```python
from build123d import *

# Parameters (mm, degrees)
F0_W     = 35
F0_H     = 20
F1_DEPTH = 5
F2_R     = 2.49999


# Not quite as in the source:
# - a fillet or chamfer is up to 0.001 mm smaller than in the source, because OpenCascade refuses the exact size


with BuildPart() as f1:
    # F0 (on Top) → F1 (new body)
    with BuildSketch(Plane.XY):
        Rectangle(F0_W, F0_H)
        Polygon((3, -1), (15, -1), (15, -6), (-15, -6), (-15, -1), (-3, -1), (-3, 5), (3, 5), align=None, mode=Mode.SUBTRACT)
    extrude(amount=F1_DEPTH)

    # F2 (radius 2.5 in the source; OpenCascade refuses exactly that, so slightly less here)
    f2_edges = [f1.edges().sort_by_distance(p)[0] for p in [
        (-17.5, -10, 2.5),
        (17.5, -10, 2.5),
        (0, -10, 0),
        (0, -10, 5),
    ]]
    fillet(f2_edges, radius=F2_R)


solid = f1.part
```
For this review, take the finished solid that the model builds, in its own axes (mm). A direction names the side the tool comes from. Round coordinates to 2 decimals unless told otherwise and drop trailing zeros. Order: outer loops, then holes, each group sorted by start corner. A loop starts at its lowest first (then second) coordinate and runs counter-clockwise, first axis right, second up.
Q1. Machinability: for faces 4 (the flat face through (-15, -4, 2)), 5 (the flat face through (-17.5, 1, 2)), which of the approach directions +Z, -Z, +X, -X, +Y, -Y give a long, thin tool a straight path to every point of the face, cutting with its end or side? Answer none if there is none.
Findings below:
face 4: +Z, -Z
face 5: +Z, -Z, -X, +Y, -Y
Q2. We need section D-D, the plane y = 1.75. Give the boundary of the cut face in (x, z).
Findings below:
outline: (-17.5, 0) - (-3, 0) - (-3, 5) - (-17.5, 5) - close; (3, 0) - (17.5, 0) - (17.5, 5) - (3, 5) - close
Q3. We need section C-C, the plane z = 4. Give the boundary of the cut face in (x, y).
Findings below:
outline: (-17.5, -7.5) arc R2.5 ccw to (-16.5, -9.5) - (16.5, -9.5) arc R2.5 ccw to (17.5, -7.5) - (17.5, 10) - (-17.5, 10) - close; hole (-15, -6) - (15, -6) - (15, -1) - (3, -1) - (3, 5) - (-3, 5) - (-3, -1) - (-15, -1) - close
Q4. Mouldability with a two-part tool opening along Y and no side actions: class faces 1 (the flat face through (-0.2, 5.3, 0)), 2 (the cylindrical face through (0.245, -9.287, 4.248)), 3 (the flat face through (-9, -1, 2)) as pulls with the +Y half, pulls with the -Y half, needs draft (parallel to the pull), parting line crosses it, or undercut.
Findings below:
face 1: needs draft
face 2: pulls with the -Y half
face 3: undercut
Q5. Insertion check: P1, Ø6, axis at x = 13.5, y = -2, coming from the -Z side. The pin has a flat end and moves straight along its axis. Give the tip position at first contact, or say it passes through.
Findings below:
P1: stops at z = 0
Q6. We need section A-A, the plane y = -1.75. Give the boundary of the cut face in (x, z), plus the area to 3 significant figures.
Findings below:
outline: (-17.5, 0) - (-15, 0) - (-15, 5) - (-17.5, 5) - close; (15, 0) - (17.5, 0) - (17.5, 5) - (15, 5) - close
area: 25.0 mm2
Q7. Wall thickness on line 1 (Y direction, x = -7, z = 2.5); line 2 (X direction, y = -0.5, z = 4.75); line 3 (X direction, y = -1.75, z = 1.4): over which ranges is each line inside the solid? List them lowest first.
Findings below:
line 1: y = -10 to -6, -1 to 10
line 2: x = -17.5 to -3, 3 to 17.5
line 3: x = -17.5 to -15, 15 to 17.5
